from build123d import *

# Parameters (mm, degrees)
EXTRUDE_1_DEPTH = 8
FILLET_1_R      = 30
FILLET_2_R      = 5


with BuildPart() as part:
    # 草图1 → 凸台-拉伸1 (new body)
    with BuildSketch(Plane.XY):
        Polygon((-25, 0), (25, 0), (50, 40), (50, 50), (-50, 50), (-50, 40), align=None)
    extrude(amount=EXTRUDE_1_DEPTH)

    # 圆角1
    fillet_1_edges = [part.edges().sort_by_distance(p)[0] for p in [
        (25, 0, 4),
        (-25, 0, 4),
    ]]
    fillet(fillet_1_edges, radius=FILLET_1_R)

    # 圆角2
    fillet_2_edges = [part.edges().sort_by_distance(p)[0] for p in [
        (50, 40, 4),
        (-50, 40, 4),
    ]]
    fillet(fillet_2_edges, radius=FILLET_2_R)


solid = part.part
Geometry: final body of the model. Coordinates: model frame, mm. Coordinates: 2 decimals unless noted, no trailing zeros. Order: outer loops, then holes, each group sorted by start corner. A loop starts at its lowest first (then second) coordinate and runs counter-clockwise, first axis right, second up.
(1) Section query A-A (z = 5). Return the cut outline in (x, y), plus the area to 3 significant figures.
(2) Section query B-B (x = -35). Return the cut outline in (y, z), plus the area to 3 significant figures.
(3) Section query C-C (y = 16). Return the cut outline in (x, z).
(4) Draft query along Y for faces 1 (the face through (49.8, 40.04, 4.06)), 2 (the face through (-1, 31, 0)), 3 (the face through (1, 50, 4)). Return one class per face: pulls with the +Y half, pulls with the -Y half, needs draft (parallel to the pull), parting line crosses it, or undercut.
(5) Material intervals for probe 1 along Y at (x, z) = (-18, 2.5); probe 2 along Y at (x, z) = (23, 2.75); probe 3 along X at (y, z) = (13, 4), sorted ascending.
Solution:
1. outline: (-50, 41.43) arc R5 ccw to (-49.24, 38.78) - (-33.81, 14.1) arc R30 ccw to (-8.37, 0) - (8.37, 0) arc R30 ccw to (33.81, 14.1) - (49.24, 38.78) arc R5 ccw to (50, 41.43) - (50, 50) - (-50, 50) - close
1. area: 3,910 mm2
2. outline: (16, 0) - (50, 0) - (50, 8) - (16, 8) - close
2. area: 272 mm2
3. outline: (-35, 0) - (35, 0) - (35, 8) - (-35, 8) - close
4. face 1: pulls with the -Y half
4. face 2: needs draft
4. face 3: pulls with the +Y half
5. probe 1: y = 1.59 to 50
5. probe 2: y = 3.81 to 50
5. probe 3: x = -33.09 to 33.09
